Verification items for the finished model (mm, model axes). A direction names the side the tool comes from. Coordinates: 2 decimals unless noted, no trailing zeros. Order: outer loops, then holes, each group sorted by start corner. A loop starts at its lowest first (then second) coordinate and runs counter-clockwise, first axis right, second up. Notation, with made-up numbers: (3.25, 76) -> (40.25, 76) arc R14 ccw to (40.25, 83) -> close; hole circle Ø5 at (48, -8.75). An arc over 180 degrees is marked (long way). Write each question's results on one line, items separated by ' | '. Start each with the question number.
(1) Go/stop test with flat-tipped pins: pin 1 (4 mm diameter, centred on x = -7.5, y = 4.5, fed in from -Z); pin 2 (5 mm diameter, centred on y = 3, z = -25, fed in from +X); pin 3 (2 mm diameter, centred on x = -12.5, y = 2.5, fed in from -Z). Record where each tip stops, or that it passes through.
(2) Cross-section at D-D on z = -2. Enter the section's corners in (x, y), and give its area (3 significant figures).
(3) Cross-section at C-C on x = -16. Enter the section's corners in (y, z).
(4) Thickness scan on probe 1 along X at (y, z) = (3.5, 15); probe 2 along X at (y, z) = (4.25, -24); probe 3 along Z at (x, y) = (-12.25, 2.25). Record the ranges inside material, lowest first. Write a range as [from, to].
(5) Cross-section at A-A on y = 8. Give the number of separate pieces and of enclosed holes in the cut face, and give its area (3 significant figures).
(6) Set-up check for faces 5 (the flat face through (-10.95, 5, -22)), 6 (the cylindrical face through (-2, 5, 19)): record each of +Z, -Z, +X, -X, +Y, -Y from which the full face is reachable in a straight line by a thin tool's end or side.
(7) Cross-section at B-B on z = 14. Enter the section's corners in (x, y).
(8) Draft check along X on faces 1 (the flat face through (-8.45, 5, -2)), 2 (the flat face through (-19, 10, -13)), 3 (the cylindrical face through (-17.996, 5.07, 16.038)), 4 (the flat face through (-29.95, 5, -13)). Enter one of: +X half, -X half, draft (parallel to the pull), parting line (faces both ways), or undercut.
```python
from build123d import *

# Parameters (mm, degrees)
BOSS_EXTRUDE1_DEPTH = 10
SKETCH3_R           = 2.25
CUT_EXTRUDE1_DEPTH  = 10
FILLET1_R           = 10
FILLET2_R           = 5


with BuildPart() as part:
    # Sketch2 → Boss-Extrude1 (new body)
    with BuildSketch(Plane(origin=(0, 0, 0), x_dir=(1, 0, 0), z_dir=(0, 1, 0))):
        Polygon((-8.45, 15), (-10.95, 15), (-10.95, 30), (-14.95, 30), (-14.95, 45), (-29.95, 45), (-29.95, -20), (0, -20), (0, -10), (-8.45, -10), align=None)
    extrude(amount=BOSS_EXTRUDE1_DEPTH)

    # Sketch3 → Cut-Extrude1 (cut)
    with BuildSketch(Plane(origin=(0, 10, 0), x_dir=(1, 0, 0), z_dir=(0, 1, 0))):
        with Locations(Location((-5, -15, 0), (0, 0, 270))):
            Circle(SKETCH3_R)
        with Locations(Location((-16, -15, 0), (0, 0, 270))):
            Circle(SKETCH3_R)
    extrude(amount=-CUT_EXTRUDE1_DEPTH, mode=Mode.SUBTRACT)

    # Fillet1
    fillet1_edges = [part.edges().sort_by_distance(p)[0] for p in [
        (-29.95, 5, 20),
        (-29.95, 5, -45),
    ]]
    fillet(fillet1_edges, radius=FILLET1_R)

    # Fillet2
    fillet2_edges = [part.edges().sort_by_distance(p)[0] for p in [
        (-14.95, 5, -45),
        (0, 5, 10),
        (0, 5, 20),
    ]]
    fillet(fillet2_edges, radius=FILLET2_R - 0.0001)  # a hair under: the kernel refuses the full size


solid = part.part
```
Results are:
1) pin 1: stops at z = -15 | pin 2: stops at x = -10.95 | pin 3: stops at z = -30
2) outline: (-29.95, 0) -> (-8.45, 0) -> (-8.45, 10) -> (-29.95, 10) -> close | area: 215 mm2
3) outline: (0, -43.07) -> (10, -43.07) -> (10, 12.75) -> (0, 12.75) -> close; (0, 17.25) -> (10, 17.25) -> (10, 20) -> (0, 20) -> close
4) probe 1: x = [-28.61, -18.25], [-13.75, -7.25], [-2.75, 0] | probe 2: x = [-29.95, -10.95] | probe 3: z = [-30, 20]
5) separate pieces: 1 | enclosed holes: 2 | area: 1,260 mm2
6) face 5: -Z, +X, +Y, -Y | face 6: +Z, +X, +Y, -Y
7) outline: (-29.12, 0) -> (-18.02, 0) -> (-18.02, 10) -> (-29.12, 10) -> close; (-13.98, 0) -> (-7.02, 0) -> (-7.02, 10) -> (-13.98, 10) -> close; (-2.98, 0) -> (-0.1, 0) -> (-0.1, 10) -> (-2.98, 10) -> close
8) face 1: +X half | face 2: draft | face 3: undercut | face 4: -X half
